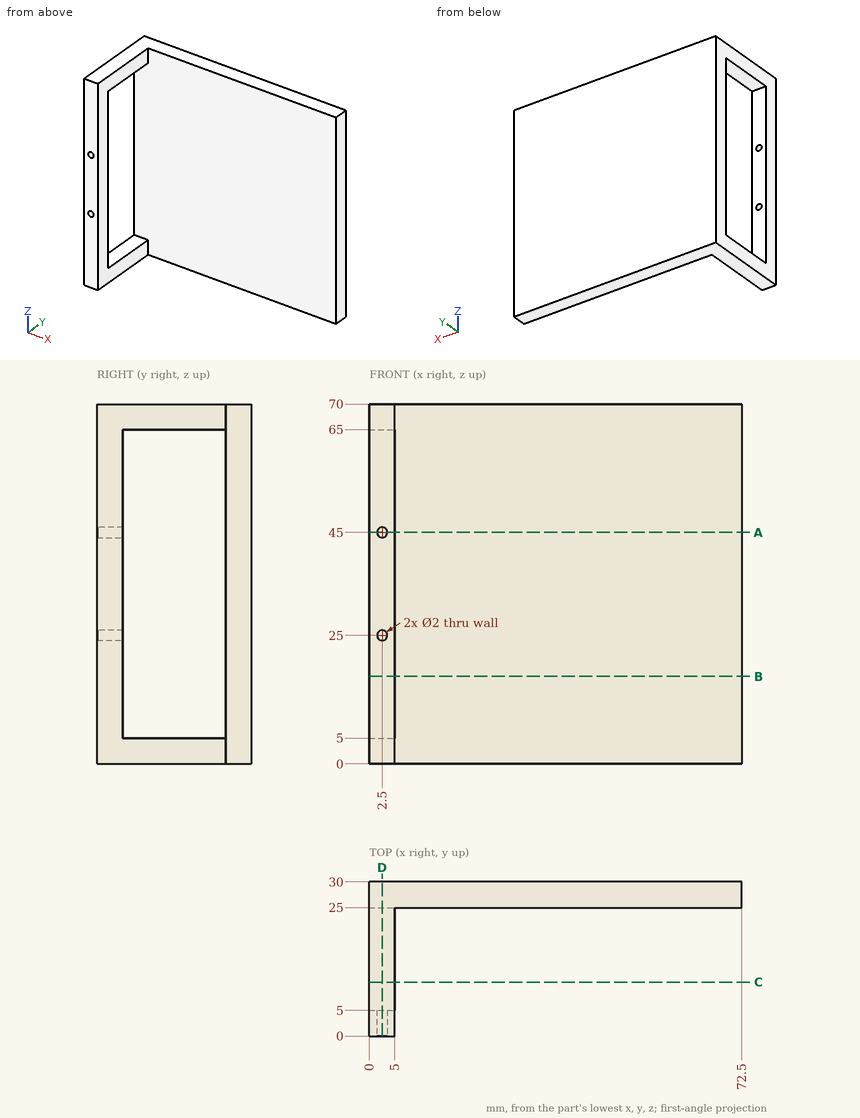
Source: three-view drawing plus pictorial views. Frame: mm from the lowest corner of the part. Give positions to 0.01 mm unless a question says otherwise; leave off trailing zeros. Write each loop counter-clockwise with the first axis right and the second up, starting at its lowest first coordinate (ties: lowest second). Pieces come first, ordered by that corner, then holes. Notation, with made-up numbers: (67.25, 6.5) -> (124.25, 6.5) arc R23 cw to (124.25, 30.5) -> close; hole circle Ø3 at (78.25, 72). An arc over 180 degrees is marked (long way). Answer in a Markdown table with one row per item.
(1) Pin query (flat end, axial travel): pin 1 (2 mm diameter, centred on x = 42.5, z = 49.5, fed in from -Y); pin 2 (12 mm diameter, centred on y = 3.5, z = 37, fed in from +X); pin 3 (12 mm diameter, centred on x = 39, y = 15.5, fed in from +Z). Return the tip coordinate at first contact, or that it passes through.
Answers below:
| item | result |
|---|---|
| pin 1 | y = 25 |
| pin 2 | x = 5 |
| pin 3 | through |
(2) Section query D-D on x = 2.5. Return loops of the section in (y, z).
Answers below:
| item | result |
|---|---|
| outline | (0, 0) -> (30, 0) -> (30, 70) -> (0, 70) -> (0, 46) -> (5, 46) -> (5, 65) -> (25, 65) -> (25, 5) -> (5, 5) -> (5, 24) -> (0, 24) -> close; (0, 26) -> (5, 26) -> (5, 44) -> (0, 44) -> close |
(3) Section query A-A on z = 45. Return loops of the section in (x, y), then the cut area to 4 significant figures.
Answers below:
| item | result |
|---|---|
| outline | (0, 0) -> (1.5, 0) -> (1.5, 5) -> (0, 5) -> close; (0, 25) -> (72.5, 25) -> (72.5, 30) -> (0, 30) -> close; (3.5, 0) -> (5, 0) -> (5, 5) -> (3.5, 5) -> close |
| area | 377.5 mm^2 |
(4) Section query C-C on y = 10.5. Return loops of the section in (x, z).
Answers below:
| item | result |
|---|---|
| outline | (0, 0) -> (5, 0) -> (5, 5) -> (0, 5) -> close; (0, 65) -> (5, 65) -> (5, 70) -> (0, 70) -> close |
(5) Section query B-B on z = 17. Return loops of the section in (x, y).
Answers below:
| item | result |
|---|---|
| outline | (0, 0) -> (5, 0) -> (5, 5) -> (0, 5) -> close; (0, 25) -> (72.5, 25) -> (72.5, 30) -> (0, 30) -> close |
(6) Ray query, line 1 along X through (y, z) = (1.95, 45); line 2 along Y through (x, z) = (44.5, 49.5); line 3 along X through (y, z) = (1.5, 22.5). Return the intervals inside material, ascending. Write a range as [from, to].
Answers below:
| item | result |
|---|---|
| line 1 | [0, 1.5], [3.5, 5] |
| line 2 | [25, 30] |
| line 3 | [0, 5] |
